The drawing under review shows one solid part. Ordinate dimensions are in mm from its lowest x, y, z. Round coordinates to 2 decimals unless told otherwise and drop trailing zeros. Loops run counter-clockwise (first coordinate to the right, second up) from the corner with the lowest first, then second, coordinate; pieces in that order, holes last. Notation, with made-up numbers: (19, 51.25) -> (41, 51.25) arc R33 cw to (41, 89.25) -> close; hole circle Ø8 at (-34, 89). An arc over 180 degrees is marked (long way). Use a Markdown table: item, result. Add a question column.
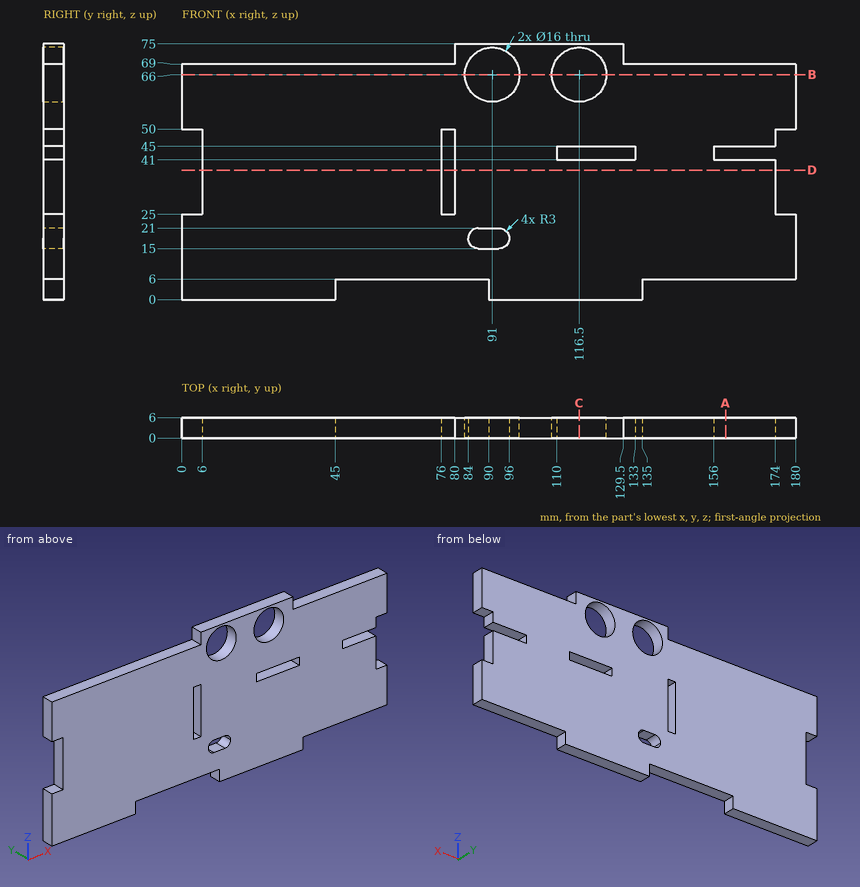
1. To check wall thickness, follow probe 1 along X at (y, z) = (3.3, 44); probe 2 along X at (y, z) = (3.8, 66); probe 3 along X at (y, z) = (5.65, 30.5). State the ranges of each line that lie inside material, in increasing order. Write a range as from..to.
2. Insertion check: P1, Ø2, axis at y = 3, z = 31, coming from the +X side; P2, Ø1.8, axis at y = 4, z = 33.5, coming from the -X side; P3, Ø3, axis at x = 148.5, y = 3.5, coming from the -Z side. Each pin has a flat end and moves straight along its axis. Give the tip position at first contact, or say it passes through.
3. Consider section A-A on x = 159.5. State the section outline as (y, z) points, plus the area to 3 significant figures.
4. Consider section B-B on z = 66. State the section outline as (x, y) points, plus the area to 3 significant figures.
5. Consider section C-C on x = 116.5. State the section outline as (y, z) points, plus the area to 3 significant figures.
6. Consider section D-D on z = 38. State the section outline as (x, y) points, plus the area to 3 significant figures.
Verdict:
| question | item | result |
|---|---|---|
| 1 | probe 1 | x = 6..76, 80..110, 133..156 |
| 1 | probe 2 | x = 0..83, 99..108.5, 124.5..180 |
| 1 | probe 3 | x = 6..76, 80..174 |
| 2 | P1 | stops at x = 174 |
| 2 | P2 | stops at x = 6 |
| 2 | P3 | stops at z = 6 |
| 3 | outline | (0, 6) -> (6, 6) -> (6, 41) -> (0, 41) -> close; (0, 45) -> (6, 45) -> (6, 69) -> (0, 69) -> close |
| 3 | area | 354 mm² |
| 4 | outline | (0, 0) -> (83, 0) -> (83, 6) -> (0, 6) -> close; (99, 0) -> (108.5, 0) -> (108.5, 6) -> (99, 6) -> close; (124.5, 0) -> (180, 0) -> (180, 6) -> (124.5, 6) -> close |
| 4 | area | 888 mm² |
| 5 | outline | (0, 0) -> (6, 0) -> (6, 41) -> (0, 41) -> close; (0, 45) -> (6, 45) -> (6, 58) -> (0, 58) -> close; (0, 74) -> (6, 74) -> (6, 75) -> (0, 75) -> close |
| 5 | area | 330 mm² |
| 6 | outline | (6, 0) -> (76, 0) -> (76, 6) -> (6, 6) -> close; (80, 0) -> (174, 0) -> (174, 6) -> (80, 6) -> close |
| 6 | area | 984 mm² |
